Geometry check sheet. Reference: the model listing, model coordinates, mm. Face numbers are marked on the shaded views. A direction names the side the tool comes from. Give positions to 0.01 mm unless a question says otherwise; leave off trailing zeros. Order: outer loops, then holes, each group sorted by start corner. A loop starts at its lowest first (then second) coordinate and runs counter-clockwise, first axis right, second up.
from build123d import *

# Parameters (mm, degrees)
F0_R     = 3.125
F1_DEPTH = 28
F2_W     = 2
F2_H     = 5.1480256068
F5_D     = 2.5
F5_DEPTH = 11.4
F5_TIP   = 0.7510757738


with BuildPart() as f1:
    # F0 (on Right) → F1 (new body)
    with BuildSketch(Plane.YZ):
        Circle(F0_R)
    extrude(amount=F1_DEPTH)

    # F2 (on Front) → F3 (revolve, cut)
    with BuildSketch(Plane.XZ):
        with Locations((2, 4.1990128034)):
            Rectangle(F2_W, F2_H)
        with Locations((6, 4.1990128034)):
            Rectangle(F2_W, F2_H)
    revolve(axis=Axis((0, 0, 0), (-1, 0, 0)), mode=Mode.SUBTRACT)

    # F5
    with Locations(Plane.YZ.offset(28)):
        with Locations((0, 0)):
            Hole(F5_D / 2, depth=F5_DEPTH)
            with Locations((0, 0, -(F5_DEPTH + F5_TIP / 2))):  # 118° drill point
                Cone(0, F5_D / 2, F5_TIP, mode=Mode.SUBTRACT)


solid = f1.part
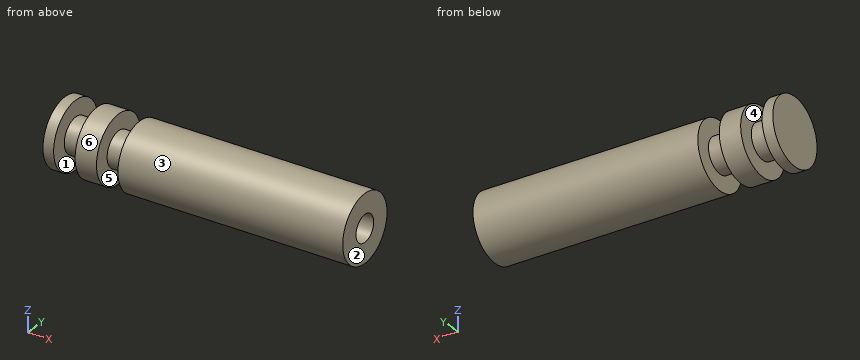
Item 1: Sectioned sample at A-A (z = -2). Enter the section's corners in (x, y), and give its area (3 significant figures).
Reported:
outline: (0, -2.4) - (1, -2.4) - (1, 2.4) - (0, 2.4) - close; (3, -2.4) - (5, -2.4) - (5, 2.4) - (3, 2.4) - close; (7, -2.4) - (28, -2.4) - (28, 2.4) - (7, 2.4) - close
area: 115 mm2
Item 2: Gauge pin test, flat ends, axial feed: pin 1 (3 mm diameter, centred on x = 12, y = -1, fed in from +Z) (3 decimals); pin 2 (1.5 mm diameter, centred on x = 6.5, z = 2.5, fed in from -Y). Record the tip position at first contact, or that the pin passes through.
Reported:
pin 1: stops at z = 3.125
pin 2: stops at y = -2.45
Item 3: Draft check along X on the marked faces 1, 2, 3 and 4. Enter one of: released by +X, released by -X, zero draft, split by the parting line, or undercut.
Reported:
face 1: undercut
face 2: released by +X
face 3: zero draft
face 4: undercut
Item 4: Set-up check for the marked faces 5 and 6: record each of +Z, -Z, +X, -X, +Y, -Y from which the full face is reachable in a straight line by a thin tool's end or side.
Reported:
face 5: none
face 6: +X, -X
Item 5: Scan lines: L1, parallel to X at y = -0.75, z = 3; L2, parallel to Z at x = 21.5, y = 0 (3 decimals). Record each from-to range of solid material in increasing order.
Reported:
L1: x = 0 to 1, 3 to 5, 7 to 28
L2: z = -3.125 to -1.25, 1.25 to 3.125
Item 6: Sectioned sample at C-C (x = 4). Enter the section's corners in (y, z) (3 decimals), and give its area (3 significant figures).
Reported:
outline: circle Ø6.25 at (0, 0)
area: 30.7 mm2
